```python
from build123d import *

# Parameters (mm, degrees)
RESSALTO_EXTRUS_O1_DEPTH = 11
ESBO_O2_W                = 12.5
ESBO_O2_H                = 2
RESSALTO_EXTRUS_O2_DEPTH = 7
RESSALTO_EXTRUS_O3_DEPTH = 7
ESBO_O4_R                = 1.95
CORTE_EXTRUS_O1_DEPTH    = 2
CORTE_EXTRUS_O2_DEPTH    = 12
CORTE_EXTRUS_O3_DEPTH    = 12


with BuildPart() as part:
    # Esboço1 → Ressalto-extrusão1 (new body)
    with BuildSketch(Plane.XY):
        with BuildLine():
            Line((-6.25, -6.25), (0, -6.25))
            ThreePointArc((0, -6.25), (-4.419417382, -4.419417382), (-6.25, 0))
            Line((-6.25, 0), (-6.25, -6.25))
        make_face()
        with BuildLine():
            Line((6.25, -6.25), (6.25, 0))
            ThreePointArc((6.25, 0), (4.419417382, -4.419417382), (0, -6.25))
            Line((0, -6.25), (6.25, -6.25))
        make_face()
        with BuildLine():
            ThreePointArc((-4.25, 0), (0, 4.25), (4.25, 0))
            Line((4.25, 0), (6.25, 0))
            ThreePointArc((6.25, 0), (4.419417387, 4.419417378), (1.3e-08, 6.25))
            ThreePointArc((1.3e-08, 6.25), (-4.419417378, 4.419417387), (-6.25, 0))
            Line((-6.25, 0), (-4.25, 0))
        make_face()
        with BuildLine():
            Line((6.25, 0), (4.25, 0))
            ThreePointArc((4.25, 0), (0, -4.25), (-4.25, 0))
            Line((-4.25, 0), (-6.25, 0))
            ThreePointArc((-6.25, 0), (-4.419417382, -4.419417382), (0, -6.25))
            ThreePointArc((0, -6.25), (4.419417382, -4.419417382), (6.25, 0))
        make_face()
    ressalto_extrus_o1 = extrude(amount=RESSALTO_EXTRUS_O1_DEPTH)

    # Esboço2 → Ressalto-extrusão2 (add)
    with BuildSketch(Plane.XY.offset(11)):
        with Locations((0, -5.25)):
            Rectangle(ESBO_O2_W, ESBO_O2_H)
    ressalto_extrus_o2 = extrude(amount=RESSALTO_EXTRUS_O2_DEPTH)

    # Esboço3 → Ressalto-extrusão3 (add)
    with BuildSketch(Plane.XY.offset(18)):
        with BuildLine():
            Line((5.25, -4.25), (6.25, -4.25))
            ThreePointArc((6.25, -4.25), (5.75, -3.75), (5.25, -4.25))
        make_face()
        with BuildLine():
            Line((-6.25, -4.25), (-5.25, -4.25))
            ThreePointArc((-5.25, -4.25), (-5.75, -3.75), (-6.25, -4.25))
        make_face()
    ressalto_extrus_o3 = extrude(amount=-RESSALTO_EXTRUS_O3_DEPTH)

    # Espelhar1: Ressalto-extrusão1, Ressalto-extrusão2, Ressalto-extrusão3 across plane
    add(ressalto_extrus_o1.mirror(Plane(origin=(0, 0, 18), x_dir=(1, 0, 0), z_dir=(0, 0, -1))))
    add(ressalto_extrus_o2.mirror(Plane(origin=(0, 0, 18), x_dir=(1, 0, 0), z_dir=(0, 0, -1))))
    add(ressalto_extrus_o3.mirror(Plane(origin=(0, 0, 18), x_dir=(1, 0, 0), z_dir=(0, 0, -1))))

    # Esboço4 → Corte-extrusão1 (cut)
    with BuildSketch(Plane(origin=(0, -4.25, 0), x_dir=(1, 0, 0), z_dir=(0, 1, 0))):
        with Locations(Location((0, -18, 0), (0, 0, 270))):
            Circle(ESBO_O4_R)
    extrude(amount=-CORTE_EXTRUS_O1_DEPTH, mode=Mode.SUBTRACT)

    # Esboço5 → Corte-extrusão2 (cut)
    with BuildSketch(Plane.XY.offset(36)):
        with BuildLine():
            Line((2.324678961, -3.557859993), (6.25, -4.25))
            Line((6.25, -4.25), (6.25, 0))
            ThreePointArc((6.25, 0), (5.958039408, 1.887926484), (5.109434749, 3.599468925))
            Line((5.109434749, 3.599468925), (3.474415629, 2.447638869))
            ThreePointArc((3.474415629, 2.447638869), (4.051466798, 1.283790009), (4.25, 0))
            ThreePointArc((4.25, 0), (3.737805879, -2.022698002), (2.324678961, -3.557859993))
        make_face()
    extrude(amount=-CORTE_EXTRUS_O2_DEPTH, mode=Mode.SUBTRACT)

    # Esboço6 → Corte-extrusão3 (cut)
    with BuildSketch(Plane(origin=(0, 0, 0), x_dir=(-1, 0, 0), z_dir=(0, 0, -1))):
        with BuildLine():
            Line((2.324678961, -3.557859993), (6.25, -4.25))
            Line((6.25, -4.25), (6.25, 0))
            ThreePointArc((6.25, 0), (5.95810098, 1.887732163), (5.10966953, 3.599135631))
            Line((5.10966953, 3.599135631), (3.474575281, 2.447412229))
            ThreePointArc((3.474575281, 2.447412229), (4.051508666, 1.283657871), (4.25, 0))
            ThreePointArc((4.25, 0), (3.737805879, -2.022698002), (2.324678961, -3.557859993))
        make_face()
    extrude(amount=-CORTE_EXTRUS_O3_DEPTH, mode=Mode.SUBTRACT)


solid = part.part
```
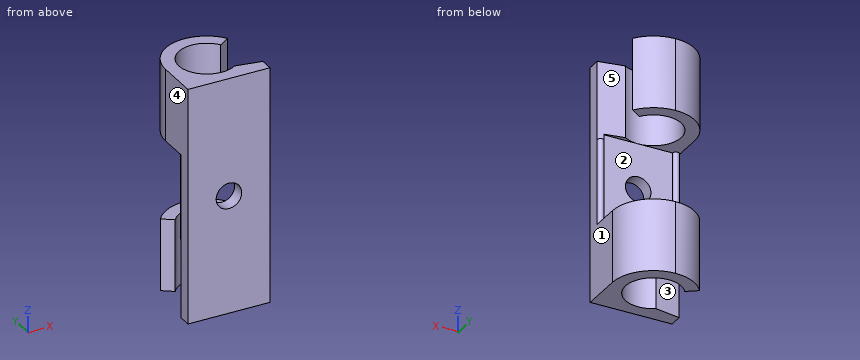
Design review of the part built by this model. Coordinates are the model's own, in mm. Face numbers are marked on the shaded views. A direction names the side the tool comes from. Give positions to 0.01 mm unless a question says otherwise; leave off trailing zeros. Loops run counter-clockwise (first coordinate to the right, second up) from the corner with the lowest first, then second, coordinate; pieces in that order, holes last. Notation, with made-up numbers: (7, 53) -> (21, 53) arc R22 cw to (21, 83) -> close; hole circle Ø7 at (-15, -3.5). An arc over 180 degrees is marked (long way). One line per item, written item: value.
Q1. For pin 1 Ø2 at (x, y) = (3, 4.5) entering from -Z; pin 2 Ø6 at (x, z) = (0, 18) entering from +Y; pin 3 Ø2 at (y, z) = (-1, 8.5) entering from -X, all flat-tipped, find the tip position at first contact; note any pin that passes through.
Numbers:
pin 1: stops at z = 0
pin 2: stops at y = -4.25
pin 3: stops at x = 3.75
Q2. We need section C-C on y = -3. Give the boundary of the cut face in (x, z), and give its area (3 significant figures).
Numbers:
outline: (-6.25, 25) -> (-3.01, 25) -> (-3.01, 36) -> (-6.25, 36) -> close; (3.01, 0) -> (6.25, 0) -> (6.25, 11) -> (3.01, 11) -> close
area: 71.3 mm^2
Q3. For L1, parallel to X at y = -5.6, z = 18; L2, parallel to Z at x = 5.25, y = 2.75; L3, parallel to X at y = 3.5, z = 2, list the stretches that pass through material, from the lowest coordinate up.
Numbers:
L1: x = -6.25 to -1.95, 1.95 to 6.25
L2: z = 0 to 11
L3: x = -4.97 to -2.41, 2.41 to 5.18
Q4. Draft analysis for pull direction Y (two halves, no side actions). For the marked faces 1, 2 and 3, state which applies: pulls with the +Y half, pulls with the -Y half, needs draft (parallel to the pull), parting line crosses it, or undercut.
Numbers:
face 1: needs draft
face 2: pulls with the +Y half
face 3: undercut
Q5. We need section B-B on x = -1.25. Give the boundary of the cut face in (y, z).
Numbers:
outline: (-6.25, 0) -> (-4.06, 0) -> (-4.06, 11) -> (-4.25, 11) -> (-4.25, 16.5) -> (-6.25, 16.5) -> close; (-6.25, 19.5) -> (-4.25, 19.5) -> (-4.25, 25) -> (-4.06, 25) -> (-4.06, 36) -> (-6.25, 36) -> close; (4.06, 0) -> (6.12, 0) -> (6.12, 11) -> (4.06, 11) -> close; (4.06, 25) -> (6.12, 25) -> (6.12, 36) -> (4.06, 36) -> close
Q6. We need section A-A on z = 18. Give the boundary of the cut face in (x, y), and give its area (3 significant figures).
Numbers:
outline: (-6.25, -6.25) -> (-1.95, -6.25) -> (-1.95, -4.25) -> (-5.25, -4.25) arc R0.5 ccw to (-6.25, -4.25) -> close; (1.95, -6.25) -> (6.25, -6.25) -> (6.25, -4.25) arc R0.5 ccw to (5.25, -4.25) -> (1.95, -4.25) -> close
area: 18.0 mm^2
Q7. We need section D-D on z = 28. Give the boundary of the cut face in (x, y).
Numbers:
outline: (-6.25, -6.25) -> (6.25, -6.25) -> (6.25, -4.25) -> (2.32, -3.56) arc R4.25 cw (long way) to (3.47, 2.45) -> (5.11, 3.6) arc R6.25 ccw to (-6.25, 0) -> close
Q8. Machinability: for the marked faces 4 and 5, which of the approach directions +Z, -Z, +X, -X, +Y, -Y give a long, thin tool a straight path to every point of the face, cutting with its end or side? Answer none if there is none.
Numbers:
face 4: +Z, -Z, -X, +Y, -Y
face 5: +Z, +X
